Read the model definition and answer for the solid it produces. Units are mm, in the model's axes. A direction names the side the tool comes from. Give positions to 0.01 mm unless a question says otherwise; leave off trailing zeros. Loops run counter-clockwise (first coordinate to the right, second up) from the corner with the lowest first, then second, coordinate; pieces in that order, holes last. Notation, with made-up numbers: (16.5, 29) - (35.5, 29) arc R13 cw to (35.5, 49) - close; hole circle Ø5 at (-12, 60). An arc over 180 degrees is marked (long way). Put each result on its own line as item: value. Start each with the question number.
1. A cutting plane is placed at A-A, the plane z = 2.15. Determine the outline of the cut face in (x, y) (3 decimals).
2. For faces 1 (the flat face through (3.175, 30, 2)), 2 (the flat face through (155.575, 30, 2)), 3 (the flat face through (2, 11.557, 2)), 4 (the flat face through (157, 11.557, 2)), determine the directions among +Z, -Z, +X, -X, +Y, -Y from which every point of the face is accessible in a straight line to the end or side of a thin tool.
3. A cutting plane is placed at B-B, the plane y = 29.5. Determine the outline of the cut face in (x, z) (3 decimals), plus the area to 3 significant figures.
4. Consider L1, parallel to X at y = 5, z = 0.9 (3 decimals); L2, parallel to X at y = 26, z = 0.3 (3 decimals). Determine where each line is inside the solid, lowest interval first. Write a range as from..to.
5. Given pin 1 Ø1.6 at (x, z) = (158, 2) entering from -Y; pin 2 Ø1 at (y, z) = (4.5, 1.5) entering from +X (3 decimals); pin 3 Ø1.6 at (x, z) = (156.5, 2.5) entering from +Y; pin 4 Ø1.7 at (x, y) = (69.58, 5.17) entering from +Z (3 decimals), each flat-ended and moving along its own axis, determine where each tip first touches the part or whether it passes through.
```python
from build123d import *

# Parameters (mm, degrees)
SKETCH1_W           = 158.75
SKETCH1_H           = 35.814
BOSS_EXTRUDE1_DEPTH = 3.175
SKETCH2_W           = 3.175
SKETCH2_H           = 11.557
CUT_EXTRUDE1_DEPTH  = 4.175
SKETCH3_R           = 1.05
CUT_EXTRUDE2_DEPTH  = 4.175


with BuildPart() as part:
    # Sketch1 → Boss-Extrude1 (new body)
    with BuildSketch(Plane.XY):
        with Locations((79.375, 17.907)):
            Rectangle(SKETCH1_W, SKETCH1_H)
    extrude(amount=BOSS_EXTRUDE1_DEPTH)

    # Sketch2 → Cut-Extrude1 (cut, through all)
    with BuildSketch(Plane.XY.offset(3.175)):
        with Locations((157.1625, 5.7785)):
            Rectangle(SKETCH2_W, SKETCH2_H)
        with Locations((1.5875, 5.7785)):
            Rectangle(SKETCH2_W, SKETCH2_H)
        with Locations((1.5875, 30.0355)):
            Rectangle(SKETCH2_W, SKETCH2_H)
        with Locations((157.1625, 30.0355)):
            Rectangle(SKETCH2_W, SKETCH2_H)
    extrude(amount=-CUT_EXTRUDE1_DEPTH, mode=Mode.SUBTRACT)

    # Sketch3 → Cut-Extrude2 (cut, through all)
    with BuildSketch(Plane(origin=(0, 0, 0), x_dir=(-1, 0, 0), z_dir=(0, 0, -1))):
        with Locations((-90.578925545, 17.471786094)):
            Circle(SKETCH3_R)
        with Locations((-69.578925545, 5.171786094)):
            Circle(SKETCH3_R)
        with Locations((-90.578925545, 5.171786094)):
            Circle(SKETCH3_R)
        with Locations((-69.578925545, 17.471786094)):
            Circle(SKETCH3_R)
    extrude(amount=-CUT_EXTRUDE2_DEPTH, mode=Mode.SUBTRACT)


solid = part.part
```
Return value:
1. outline: (0, 11.557) - (3.175, 11.557) - (3.175, 0) - (155.575, 0) - (155.575, 11.557) - (158.75, 11.557) - (158.75, 24.257) - (155.575, 24.257) - (155.575, 35.814) - (3.175, 35.814) - (3.175, 24.257) - (0, 24.257) - close; hole circle Ø2.1 at (69.579, 5.172); hole circle Ø2.1 at (69.579, 17.472); hole circle Ø2.1 at (90.579, 5.172); hole circle Ø2.1 at (90.579, 17.472)
2. face 1: +Z, -Z, -X, +Y
2. face 2: +Z, -Z, +X, +Y
2. face 3: +Z, -Z, -X, -Y
2. face 4: +Z, -Z, +X, -Y
3. outline: (3.175, 0) - (155.575, 0) - (155.575, 3.175) - (3.175, 3.175) - close
3. area: 484 mm2
4. L1: x = 3.175..68.543, 70.615..89.543, 91.615..155.575
4. L2: x = 3.175..155.575
5. pin 1: stops at y = 11.56
5. pin 2: stops at x = 155.575
5. pin 3: stops at y = 24.26
5. pin 4: passes through
